Autodesk Inventor part; units mm, degrees
ref_plane "YZ Plane" through (0, 0, 0) normal (1, 0, 0) x (0, 1, 0)
ref_plane "XZ Plane" through (0, 0, 0) normal (0, 1, 0) x (-1, 0, 0)
ref_plane "XY Plane" through (0, 0, 0) normal (0, 0, 1) x (1, 0, 0)
sketch "Sketch1" plane through (0, 0, 0) normal (0, 1, 0) x (-1, 0, 0)
  line L0 (0, 0) -> (37.465, 0)
  line L1 (37.465, 0) -> (37.465, -48.641)
  line L2 (37.465, -48.641) -> (0, -48.641)
  line L3 (0, -48.641) -> (0, 0)
  line L4 (4.2291, -4.2291) -> (34.5059, -4.2291)
  line L5 (34.5059, -4.2291) -> (34.5059, -45.6819)
  line L6 (34.5059, -45.6819) -> (4.2291, -45.6819)
  line L7 (4.2291, -45.6819) -> (4.2291, -4.2291)
  line L8 (4.2291, -4.2291) -> (34.5059, -45.6819) construction
  line L9 (34.5059, -4.2291) -> (4.2291, -45.6819) construction
  point P0 (19.3675, -24.9555)
  dimension "d0" = 37.465
  dimension "d1" = 48.641
  dimension "d2" = 30.2768
  dimension "d3" = 41.4528
extrude "Extrusion1" add sketch "Sketch1" along normal blind 2.54 contours L4 L5 L6 L7
extrude "Extrusion2" add sketch "Sketch1" along normal blind 1.778
properties part number "Valve Holder-3valve-withwirebox-lidforbox"
Here's how the part is built. I have some questions about the finished solid (model axes, mm). Coordinates: 2 decimals unless noted, no trailing zeros. Order: outer loops, then holes, each group sorted by start corner. A loop starts at its lowest first (then second) coordinate and runs counter-clockwise, first axis right, second up.
Item 1: I need wall thicknesses on probe 1 along Z at (x, y) = (-8, 2.15); probe 2 along Y at (x, z) = (-31.5, -3); probe 3 along X at (y, z) = (2.2, -41.5). Which ranges of each line are inside material? Lowest first, please.
Response values:
probe 1: z = -45.68 to -4.23
probe 2: y = 0 to 1.78
probe 3: x = -34.51 to -4.23
Item 2: I'm going to push a flat-ended pin straight in: pin 1 Ø0.6 at (y, z) = (2.5, -30.5) entering from +X. Where does the tip first touch, or does it pass through?
Response values:
pin 1: stops at x = -4.23
Item 3: If we section it at B-B, the plane x = -29: List the corners of the cut face in (y, z) for me.
Response values:
outline: (0, -48.64) - (1.78, -48.64) - (1.78, -45.68) - (2.54, -45.68) - (2.54, -4.23) - (1.78, -4.23) - (1.78, 0) - (0, 0) - close
Item 4: If we section it at A-A, the plane z = -17: List the corners of the cut face in (x, y) for me (3 decimals), then the cut area to 3 significant figures.
Response values:
outline: (-37.465, 0) - (0, 0) - (0, 1.778) - (-4.229, 1.778) - (-4.229, 2.54) - (-34.506, 2.54) - (-34.506, 1.778) - (-37.465, 1.778) - close
area: 89.7 mm2
